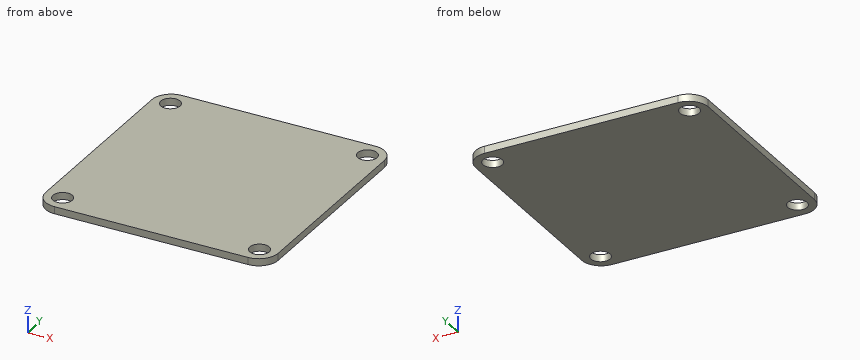
from build123d import *

# Parameters (mm, degrees)
F0_W     = 36
F0_H     = 36
F1_DEPTH = 1.1
F3_D     = 3
F4_R     = 3


with BuildPart() as f1:
    # F0 (on Top) → F1 (new body)
    with BuildSketch(Plane.XY):
        with Locations((18, 18)):
            Rectangle(F0_W, F0_H)
    extrude(amount=F1_DEPTH)

    # F3 (through all)
    with Locations(Plane.XY.offset(1.1)):
        with Locations((2.75, 33.25), (33.25, 33.25), (2.75, 2.75), (33.25, 2.75)):
            Hole(F3_D / 2)

    # F4
    f4_edges = [f1.edges().sort_by_distance(p)[0] for p in [
        (36, 0, 0.55),
        (0, 0, 0.55),
        (0, 36, 0.55),
        (36, 36, 0.55),
    ]]
    fillet(f4_edges, radius=F4_R)


solid = f1.part
For this review, take the finished solid that the model builds, in its own axes (mm). Round coordinates to 2 decimals unless told otherwise and drop trailing zeros. Order: outer loops, then holes, each group sorted by start corner. A loop starts at its lowest first (then second) coordinate and runs counter-clockwise, first axis right, second up. Notation, with made-up numbers: M -28.75,46 L -7.75,46 A18 ccw -7.75,54 Z; hole C 61,10 d1. An arc over 180 degrees is marked long. Use a Markdown table: item, result. Add a question column.
Item 1: Add section A-A, the plane z = 0.6. Give the boundary of the cut face in (x, y).
Item 2: To check wall thickness, follow line 1 along Y through (x, z) = (2.75, 0.7); line 2 along X through (y, z) = (33.5, 0.7); line 3 along X through (y, z) = (32.5, 0.85). State the ranges of each line that lie inside material, in increasing order.
Item 3: Insertion check: pin 1 (2.5 mm diameter, centred on x = 33.25, y = 2.75, fed in from +Z). The pin has a flat end and moves straight along its axis. Give the tip position at first contact, or say it passes through.
Geometry results:
| question | item | result |
|---|---|---|
| 1 | outline | M 0,3 A3 ccw 3,0 L 33,0 A3 ccw 36,3 L 36,33 A3 ccw 33,36 L 3,36 A3 ccw 0,33 Z; hole C 2.75,2.75 d3; hole C 2.75,33.25 d3; hole C 33.25,2.75 d3; hole C 33.25,33.25 d3 |
| 2 | line 1 | y = 0.01 to 1.25, 4.25 to 31.75, 34.75 to 35.99 |
| 2 | line 2 | x = 0.04 to 1.27, 4.23 to 31.77, 34.73 to 35.96 |
| 2 | line 3 | x = 0 to 1.45, 4.05 to 31.95, 34.55 to 36 |
| 3 | pin 1 | passes through |
